from build123d import *

# Parameters (mm, degrees)
CUT_EXTRUDE1_DEPTH = 0.5
CHAMFER1_SIZE      = 0.5
CHAMFER1_SIZE_2    = 0.866025404
FILLET1_R          = 0.25
FILLET2_R          = 0.1
FILLET3_R          = 0.25
CHAMFER2_SIZE      = 0.25


with BuildPart() as part:
    # Sketch1 → Revolve1 (revolve)
    with BuildSketch(Plane.XY):
        Polygon((0, 0), (3, 0), (3, -1), (1.25, -1), (1.25, -4.5), (0, -4.5), align=None)
    revolve(axis=Axis((0, -217.245924753, 0), (0, 1, 0)))

    # Sketch2 → Cut-Extrude1 (cut)
    with BuildSketch(Plane(origin=(0, 0, 0), x_dir=(1, 0, 0), z_dir=(0, 1, 0))):
        Polygon((-0.5, 0.5), (-0.5, 1.5), (0.5, 1.5), (0.5, 0.5), (1.5, 0.5), (1.5, -0.5), (0.5, -0.5), (0.5, -1.5), (-0.5, -1.5), (-0.5, -0.5), (-1.5, -0.5), (-1.5, 0.5), align=None)
    extrude(amount=-CUT_EXTRUDE1_DEPTH, mode=Mode.SUBTRACT)

    # Chamfer1
    # the kernel refuses this chamfer: 0.866025404, 0.5 mm, written as the material it adds along each edge
    with BuildSketch(Plane(origin=(-1.5, -0.5, 0.5), x_dir=(-0.0578938624026749, 0.9983227437537924, 0), z_dir=(0, 0, -1)), Plane(origin=(0.5, -0.5, 1.5), x_dir=(-3.4244955923263397e-15, 0.9983227437537926, 0.057893862402671484), z_dir=(-1, 0, 0)), Plane(origin=(1.5, -0.5, -0.5), x_dir=(0.057893862402667626, 0.9983227437537928, 0), z_dir=(0, 0, 1)), Plane(origin=(-0.5, -0.5, -1.5), x_dir=(-3.4244955923263397e-15, 0.9983227437537926, -0.057893862402671484), z_dir=(1, 0, 0))) as chamfer1_piece_1:
        Polygon((CHAMFER1_SIZE * 0.998322743754, CHAMFER1_SIZE * 0.0578938624027), (-CHAMFER1_SIZE_2 * 0.0578938623883, CHAMFER1_SIZE_2 * 0.998322743505), (0, 0), align=None)
    extrude(amount=1)

    # Fillet1
    # the kernel refuses this fillet: 0.25 mm, written as the material it takes off along each edge
    with BuildSketch(Plane(origin=(-0.5, 0.625, 0.5), x_dir=(-1, 0, 0), z_dir=(0, -1, 0))) as fillet1_piece_1_section:
        with BuildLine():
            CenterArc((FILLET1_R, -FILLET1_R), FILLET1_R, 90, 90)
            Line((0, -FILLET1_R), (0, 0))
            Line((0, 0), (FILLET1_R, 0))
        make_face()
    fillet1_piece_1 = extrude(amount=1.125, mode=Mode.PRIVATE)
    fillet1_piece_1 = split(fillet1_piece_1, bisect_by=Plane(origin=(-0.82036424, -0.392387889, 0.556422311), z_dir=(0.4999999999999566, 0.8660254037844637, 0)), keep=Keep.TOP, mode=Mode.PRIVATE)
    fillet1_piece_1 = split(fillet1_piece_1, bisect_by=Plane(origin=(-0.556422311, -0.392387889, 0.82036424), z_dir=(0, 0.8660254037844637, -0.4999999999999566)), keep=Keep.TOP, mode=Mode.PRIVATE)
    add(fillet1_piece_1, mode=Mode.SUBTRACT)
    with BuildSketch(Plane(origin=(-0.5, 0.625, -0.5), x_dir=(-1, 0, 0), z_dir=(0, -1, 0))) as fillet1_piece_2_section:
        with BuildLine():
            CenterArc((FILLET1_R, FILLET1_R), FILLET1_R, 180, 90)
            Line((0, FILLET1_R), (0, 0))
            Line((0, 0), (FILLET1_R, 0))
        make_face()
    fillet1_piece_2 = extrude(amount=1.125, mode=Mode.PRIVATE)
    fillet1_piece_2 = split(fillet1_piece_2, bisect_by=Plane(origin=(-0.82036424, -0.392387889, -0.556422311), z_dir=(0.4999999999999566, 0.8660254037844637, 0)), keep=Keep.TOP, mode=Mode.PRIVATE)
    fillet1_piece_2 = split(fillet1_piece_2, bisect_by=Plane(origin=(-0.556422311, -0.392387889, -0.82036424), z_dir=(0, 0.8660254037844637, 0.4999999999999566)), keep=Keep.TOP, mode=Mode.PRIVATE)
    add(fillet1_piece_2, mode=Mode.SUBTRACT)
    with BuildSketch(Plane(origin=(0.5, 0.625, 0.5), x_dir=(1, 0, 0), z_dir=(0, -1, 0))) as fillet1_piece_3_section:
        with BuildLine():
            CenterArc((FILLET1_R, FILLET1_R), FILLET1_R, 180, 90)
            Line((0, FILLET1_R), (0, 0))
            Line((0, 0), (FILLET1_R, 0))
        make_face()
    fillet1_piece_3 = extrude(amount=1.125, mode=Mode.PRIVATE)
    fillet1_piece_3 = split(fillet1_piece_3, bisect_by=Plane(origin=(0.82036424, -0.392387889, 0.556422311), z_dir=(-0.4999999999999566, 0.8660254037844637, 0)), keep=Keep.TOP, mode=Mode.PRIVATE)
    fillet1_piece_3 = split(fillet1_piece_3, bisect_by=Plane(origin=(0.556422311, -0.392387889, 0.82036424), z_dir=(0, 0.8660254037844637, -0.4999999999999566)), keep=Keep.TOP, mode=Mode.PRIVATE)
    add(fillet1_piece_3, mode=Mode.SUBTRACT)
    with BuildSketch(Plane(origin=(0.5, 0.625, -0.5), x_dir=(0, 0, -1), z_dir=(0, -1, 0))) as fillet1_piece_4_section:
        with BuildLine():
            CenterArc((FILLET1_R, FILLET1_R), FILLET1_R, 180, 90)
            Line((0, FILLET1_R), (0, 0))
            Line((0, 0), (FILLET1_R, 0))
        make_face()
    fillet1_piece_4 = extrude(amount=1.125, mode=Mode.PRIVATE)
    fillet1_piece_4 = split(fillet1_piece_4, bisect_by=Plane(origin=(0.556422311, -0.392387889, -0.82036424), z_dir=(0, 0.8660254037844637, 0.4999999999999566)), keep=Keep.TOP, mode=Mode.PRIVATE)
    fillet1_piece_4 = split(fillet1_piece_4, bisect_by=Plane(origin=(0.82036424, -0.392387889, -0.556422311), z_dir=(-0.4999999999999566, 0.8660254037844637, 0)), keep=Keep.TOP, mode=Mode.PRIVATE)
    add(fillet1_piece_4, mode=Mode.SUBTRACT)

    # Fillet2
    fillet2_edges = [part.edges().sort_by_distance(p)[0] for p in [
        (-1.5, 0, 0),
        (-1.125, 0, 0.5),
        (0, 0, 1.5),
        (0.5, 0, 1.125),
        (1.5, 0, 0),
        (1.125, 0, -0.5),
        (0, 0, -1.5),
        (-0.5, 0, -1.125),
        (-0.5, 0, 1.125),
        (-1.125, 0, -0.5),
        (0.5, 0, -1.125),
        (1.125, 0, 0.5),
        (0.573223305, 0, -0.573223305),
        (0.573223305, 0, 0.573223305),
        (-0.573223305, 0, -0.573223305),
        (-0.573223305, 0, 0.573223305),
    ]]
    fillet(fillet2_edges, radius=FILLET2_R)

    # Fillet3
    fillet3_edges = [part.edges().sort_by_distance(p)[0] for p in [
        (-3, -1, 0),
        (-3, 0, 0),
    ]]
    fillet(fillet3_edges, radius=FILLET3_R)

    # Chamfer2
    chamfer2_edges = [part.edges().sort_by_distance(p)[0] for p in [
        (-1.25, -4.5, 0),
    ]]
    chamfer(chamfer2_edges, length=CHAMFER2_SIZE)


solid = part.part
Design review of the part built by this model. Coordinates are the model's own, in mm. A direction names the side the tool comes from. Coordinates: 2 decimals unless noted, no trailing zeros. Order: outer loops, then holes, each group sorted by start corner. A loop starts at its lowest first (then second) coordinate and runs counter-clockwise, first axis right, second up.
Item 1: For pin 1 Ø1.5 at (x, z) = (-2, 1.5) entering from -Y; pin 2 Ø1.5 at (y, z) = (-1, -1) entering from +X; pin 3 Ø2 at (y, z) = (-4, 1) entering from +X, all flat-tipped, find the tip position at first contact; note any pin that passes through.
Item 2: Take a section at B-B, the plane z = 0. Write out the cut boundary in (x, y).
Item 3: The part is to be moulded in two halves that separate along X. For faces 4 (the flat face through (1, -1, 1)), 5 (the cylindrical face through (-3, -0.5, -0.1)), 6 (the flat face through (1.061, -0.253, -0.008)), say which applies: pulls with the +X half, pulls with the -X half, needs draft (parallel to the pull), parting line crosses it, or undercut.
Item 4: Take a section at D-D, the plane y = -2.25. Write out the cut boundary in (x, z), then the cut area to 3 significant figures.
Item 5: For faces 1 (the flat face through (1, 0, -1)), 2 (the flat face through (0.008, -0.253, 1.061)), 3 (the cylindrical face through (-0.27, -2.65, 1.22)), list the 3-axis set-ups (+Z, -Z, +X, -X, +Y, -Y) from which the entire face can be reached by the end or side of a thin tool; tool diameter is ignored.
Item 6: Take a section at C-C, the plane y = -0.65. Write out the cut boundary in (x, z).
Item 7: Take a section at A-A, the plane x = 0. Write out the cut boundary in (y, z), then the cut area to 3 significant figures.
Item 8: For line 1 (X direction, y = -2.4, z = 1); line 2 (Y direction, x = 2.25, z = 0.75); line 3 (X direction, y = -2.2, z = 0.75), list the stretches that pass through material, from the lowest coordinate up.
The answers:
1. pin 1: stops at y = -1
1. pin 2: stops at x = 2.99
1. pin 3: stops at x = 1.25
2. outline: (-3, -0.75) arc R0.25 ccw to (-2.75, -1) - (-1.25, -1) - (-1.25, -4.25) - (-1, -4.5) - (1, -4.5) - (1.25, -4.25) - (1.25, -1) - (2.75, -1) arc R0.25 ccw to (3, -0.75) - (3, -0.25) arc R0.25 ccw to (2.75, 0) - (1.53, 0) arc R0.1 ccw to (1.48, -0.01) - (0.63, -0.5) - (-0.63, -0.5) - (-1.48, -0.01) arc R0.1 ccw to (-1.53, 0) - (-2.75, 0) arc R0.25 ccw to (-3, -0.25) - close
3. face 4: needs draft
3. face 5: parting line crosses it
3. face 6: undercut
4. outline: circle Ø2.5 at (0, 0)
4. area: 4.91 mm2
5. face 1: +Z, -Z, +X, -X, +Y
5. face 2: +Y
5. face 3: -Y
6. outline: circle Ø6 at (0, 0)
7. outline: (-4.5, -1) - (-4.25, -1.25) - (-1, -1.25) - (-1, -2.75) arc R0.25 ccw to (-0.75, -3) - (-0.25, -3) arc R0.25 ccw to (0, -2.75) - (0, -1.53) arc R0.1 ccw to (-0.01, -1.48) - (-0.5, -0.63) - (-0.5, 0.63) - (-0.01, 1.48) arc R0.1 ccw to (0, 1.53) - (0, 2.75) arc R0.25 ccw to (-0.25, 3) - (-0.75, 3) arc R0.25 ccw to (-1, 2.75) - (-1, 1.25) - (-4.25, 1.25) - (-4.5, 1) - close
7. area: 13.6 mm2
8. line 1: x = -0.75 to 0.75
8. line 2: y = -1 to 0
8. line 3: x = -1 to 1
